```python
from build123d import *

# Parameters (mm, degrees)
SKETCH1_R           = 2
BOSS_EXTRUDE2_DEPTH = 2
CUT_EXTRUDE2_DEPTH  = 9
CUT_EXTRUDE3_DEPTH  = 9
CUT_EXTRUDE4_DEPTH  = 10
CUT_EXTRUDE5_DEPTH  = 10
CUT_EXTRUDE6_DEPTH  = 10
CUT_EXTRUDE8_DEPTH  = 20


with BuildPart() as part:
    # Sketch1 → Boss-Extrude2 (new body)
    with BuildSketch(Plane(origin=(0, 0, 0), x_dir=(1, 0, 0), z_dir=(0, 1, 0))):
        with BuildLine():
            Line((0, 48.412862342), (0, 37.692030173))
            ThreePointArc((0, 37.692030173), (0.292893219, 36.984923392), (1, 36.692030173))
            Line((1, 36.692030173), (31.48, 36.692030173))
            Line((31.48, 36.692030173), (43.036527631, 36.692030173))
            Line((43.036527631, 36.692030173), (43.036527631, -13.307969827))
            Line((43.036527631, -13.307969827), (38.310297741, -17.310739702))
            Line((38.310297741, -17.310739702), (34.253582629, -17.310739702))
            Line((34.253582629, -17.310739702), (36, -19.267392345))
            Line((36, -19.267392345), (30.071702425, -24.288225334))
            Line((30.071702425, -24.288225334), (54.200832168, -12.602889922))
            Line((54.200832168, -12.602889922), (54.200832168, 10.267562985))
            Line((54.200832168, 10.267562985), (54.200832168, 49.412862342))
            Line((54.200832168, 49.412862342), (41.48, 49.412862342))
            Line((41.48, 49.412862342), (1, 49.412862342))
            ThreePointArc((1, 49.412862342), (0.292893219, 49.119969123), (0, 48.412862342))
        make_face()
        with Locations((45.48, 41.700609081)):
            Circle(SKETCH1_R, mode=Mode.SUBTRACT)
        with BuildLine():
            Line((15, 43.700609081), (4.549516448, 43.700609081))
            Line((4.549516448, 43.700609081), (4.549516448, 39.700609081))
            Line((4.549516448, 39.700609081), (15, 39.700609081))
            ThreePointArc((15, 39.700609081), (17, 41.700609081), (15, 43.700609081))
        make_face(mode=Mode.SUBTRACT)
    extrude(amount=BOSS_EXTRUDE2_DEPTH)

    # Sketch6 → Cut-Extrude2 (cut)
    with BuildSketch(Plane(origin=(0, 2, 0), x_dir=(1, 0, 0), z_dir=(0, 1, 0))):
        Polygon((36, -19.267392345), (38.310297741, -17.310739702), (34.253582629, -17.310739702), align=None)
    extrude(amount=-CUT_EXTRUDE2_DEPTH, mode=Mode.SUBTRACT)

    # Sketch8 → Cut-Extrude3 (cut)
    with BuildSketch(Plane(origin=(0, 2, 0), x_dir=(1, 0, 0), z_dir=(0, 1, 0))):
        Polygon((43.036527631, 36.692030173), (45.036527631, 36.692030173), (45.036527631, -11.115496155), (45.036527631, -11.614116599), (43.036527631, -13.307969827), align=None)
    extrude(amount=-CUT_EXTRUDE3_DEPTH, mode=Mode.SUBTRACT)

    # Sketch9 → Cut-Extrude4 (cut)
    with BuildSketch(Plane(origin=(0, 2, 0), x_dir=(1, 0, 0), z_dir=(0, 1, 0))):
        with BuildLine():
            Line((0, 46.692030173), (54.200832168, 46.692030173))
            Line((54.200832168, 46.692030173), (54.200832168, 49.412862342))
            Line((54.200832168, 49.412862342), (1, 49.412862342))
            ThreePointArc((1, 49.412862342), (0.292893219, 49.119969123), (0, 48.412862342))
            Line((0, 48.412862342), (0, 46.692030173))
        make_face()
    extrude(amount=-CUT_EXTRUDE4_DEPTH, mode=Mode.SUBTRACT)

    # Sketch11 → Cut-Extrude5 (cut)
    with BuildSketch(Plane(origin=(0, 2, 0), x_dir=(1, 0, 0), z_dir=(0, 1, 0))):
        with BuildLine():
            Line((1, 46.692030173), (0, 46.692030173))
            Line((0, 46.692030173), (0, 45.692030173))
            ThreePointArc((0, 45.692030173), (0.292893219, 46.399136955), (1, 46.692030173))
        make_face()
    extrude(amount=-CUT_EXTRUDE5_DEPTH, mode=Mode.SUBTRACT)

    # Sketch12 → Cut-Extrude6 (cut)
    with BuildSketch(Plane(origin=(0, 2, 0), x_dir=(1, 0, 0), z_dir=(0, 1, 0))):
        with BuildLine():
            Line((1.549516448, 36.692030173), (1.549516448, 41.700609081))
            Line((1.549516448, 41.700609081), (1.549516448, 46.692030173))
            Line((1.549516448, 46.692030173), (1, 46.692030173))
            ThreePointArc((1, 46.692030173), (0.292893219, 46.399136955), (0, 45.692030173))
            Line((0, 45.692030173), (0, 37.692030173))
            ThreePointArc((0, 37.692030173), (0.292893219, 36.984923392), (1, 36.692030173))
            Line((1, 36.692030173), (1.549516448, 36.692030173))
        make_face()
    extrude(amount=-CUT_EXTRUDE6_DEPTH, mode=Mode.SUBTRACT)

    # Sketch13 → Cut-Extrude8 (cut)
    with BuildSketch(Plane(origin=(0, 2, 0), x_dir=(1, 0, 0), z_dir=(0, 1, 0))):
        with BuildLine():
            ThreePointArc((2.549516448, 36.692030173), (1.842409666, 36.984923392), (1.549516448, 37.692030173))
            Line((1.549516448, 37.692030173), (1.549516448, 36.692030173))
            Line((1.549516448, 36.692030173), (2.549516448, 36.692030173))
        make_face()
        with BuildLine():
            Line((2.549516448, 46.692030173), (1.549516448, 46.692030173))
            Line((1.549516448, 46.692030173), (1.549516448, 45.692030173))
            ThreePointArc((1.549516448, 45.692030173), (1.842409666, 46.399136955), (2.549516448, 46.692030173))
        make_face()
    extrude(amount=-CUT_EXTRUDE8_DEPTH, mode=Mode.SUBTRACT)


solid = part.part
```
For this review, take the finished solid that the model builds, in its own axes (mm). A direction names the side the tool comes from. Coordinates: 2 decimals unless noted, no trailing zeros. Order: outer loops, then holes, each group sorted by start corner. A loop starts at its lowest first (then second) coordinate and runs counter-clockwise, first axis right, second up. Notation, with made-up numbers: (25, 12) -> (53, 12) arc R18 ccw to (53, 22) -> close; hole circle Ø3 at (-21, 74.5). An arc over 180 degrees is marked (long way). Use CSV: the item, a comma, the result in double quotes. Start each with the question number.
Item 1: Insertion check: pin 1 (1 mm diameter, centred on y = 0.5, z = -2, fed in from -X); pin 2 (1 mm diameter, centred on x = 7.5, y = 1.5, fed in from +Z). Each pin has a flat end and moves straight along its axis. Give the tip position at first contact, or say it passes through.
Item 2: We need section A-A, the plane x = 6. Give the boundary of the cut face in (y, z), then the cut area to 3 significant figures.
Item 3: We need section C-C, the plane x = 39.5. Give the boundary of the cut face in (y, z).
Item 4: We need section B-B, the plane y = 1.2. Give the boundary of the cut face in (x, z).
Item 5: We need section D-D, the plane z = -9. Give the boundary of the cut face in (x, y).
Item 6: Draft analysis for pull direction X (two halves, no side actions). For faces 1 (the face through (45.037, 1, -12)), 2 (the face through (54.201, 1, -17)), 3 (the face through (45.3, 0, -21.9)), 4 (the face through (46.403, 0.986, -39.926)), state which applies: pulls with the +X half, pulls with the -X half, needs draft (parallel to the pull), parting line crosses it, or undercut.
Item 7: For faces 5 (the face through (23, 1, -36.692)), 6 (the face through (10, 1, -43.701)), 7 (the face through (41.967, 0.986, 18.527)), list the 3-axis set-ups (+Z, -Z, +X, -X, +Y, -Y) from which the entire face can be reached by the end or side of a thin tool; tool diameter is ignored.
Item 8: Wall thickness on probe 1 along Z at (x, y) = (13.5, 1.15); probe 2 along X at (y, z) = (0.9, 9.5); probe 3 along Z at (x, y) = (45.48, 1.3): over which ranges is each line inside the solid? List them lowest first.
Derived:
1,pin 1,"stops at x = 45.04"
1,pin 2,"stops at z = -36.69"
2,outline,"(0, -46.69) -> (2, -46.69) -> (2, -43.7) -> (0, -43.7) -> close; (0, -39.7) -> (2, -39.7) -> (2, -36.69) -> (0, -36.69) -> close"
2,area,"12.0 mm^2"
3,outline,"(0, -46.69) -> (2, -46.69) -> (2, -36.69) -> (0, -36.69) -> close; (0, 16.3) -> (2, 16.3) -> (2, 19.72) -> (0, 19.72) -> close"
4,outline,"(1.55, -45.69) arc R1 ccw to (2.55, -46.69) -> (54.2, -46.69) -> (54.2, 12.6) -> (30.07, 24.29) -> (45.04, 11.61) -> (45.04, -36.69) -> (2.55, -36.69) arc R1 ccw to (1.55, -37.69) -> close; hole (4.55, -43.7) -> (15, -43.7) arc R2 ccw to (15, -39.7) -> (4.55, -39.7) -> close; hole circle Ø4 at (45.48, -41.7)"
5,outline,"(45.04, 0) -> (54.2, 0) -> (54.2, 2) -> (45.04, 2) -> close"
6,face 1,"pulls with the -X half"
6,face 2,"pulls with the +X half"
6,face 3,"needs draft"
6,face 4,"undercut"
7,face 5,"-X, +Y, -Y"
7,face 6,"+Y, -Y"
7,face 7,"+Z, +X, +Y, -Y"
8,probe 1,"z = -46.69 to -43.7, -39.7 to -36.69"
8,probe 2,"x = 45.04 to 54.2"
8,probe 3,"z = -46.69 to -43.7, -39.7 to 16.83"
